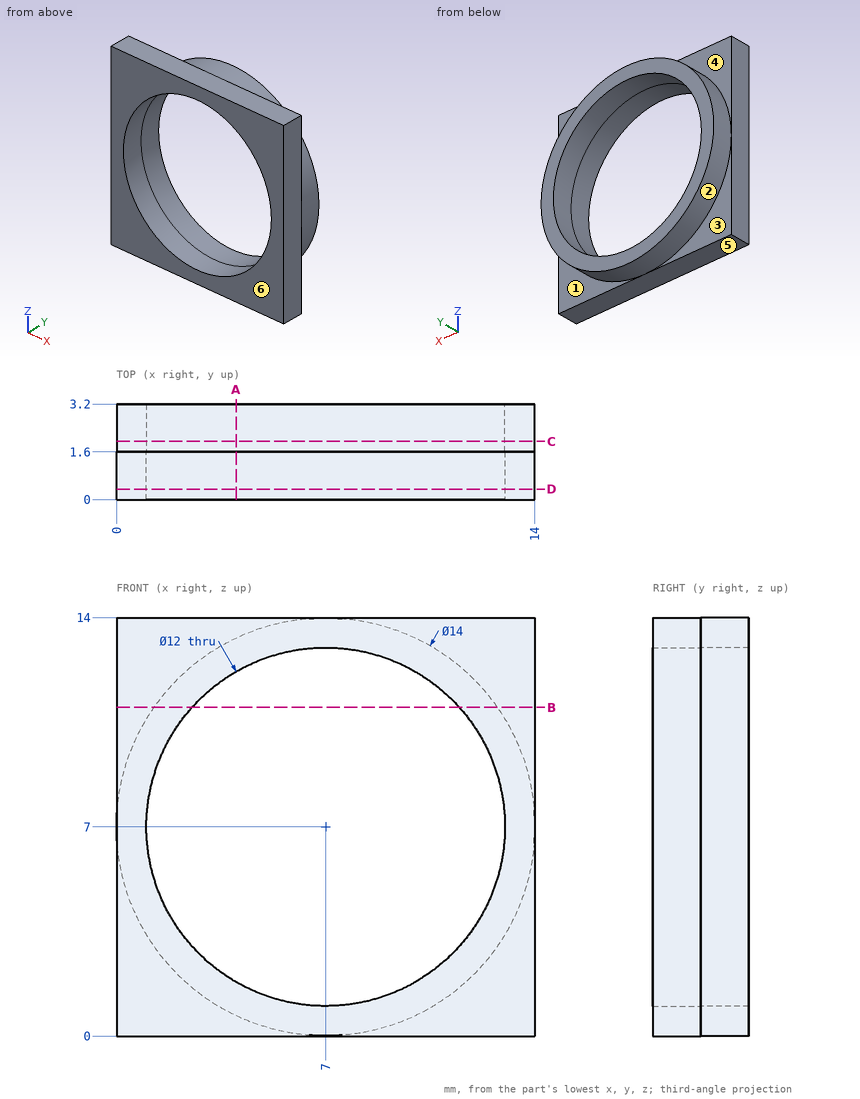
For this review, use the dimensioned drawing (mm, ordinates from the lowest corner) and the shaded views. A direction names the side the tool comes from. Coordinates: 2 decimals unless noted, no trailing zeros. Loops run counter-clockwise (first coordinate to the right, second up) from the corner with the lowest first, then second, coordinate; pieces in that order, holes last. Notation, with made-up numbers: (5, 23) - (10, 23) arc R3 ccw to (10, 28) - close; hole circle Ø3 at (53.5, -9). An arc over 180 degrees is marked (long way). Use one line per item in the form item = value. Start each with the question number.
1) Take a section at A-A (x = 4). State the section outline as (y, z) points, plus the area to 3 significant figures.
2) Take a section at D-D (y = 0.35). State the section outline as (x, z) points, plus the area to 3 significant figures.
3) Draft analysis for pull direction Y (two halves, no side actions). For the marked faces 4, 5 and 6, state which applies: released by +Y, released by -Y, zero draft, split by the parting line, or undercut.
4) For pin 1 (1 mm diameter, centred on y = 2.5, z = 8.5, fed in from -X); pin 2 (7 mm diameter, centred on x = 7, z = 7, fed in from +Y), all flat-tipped, find the tip position at first contact; note any pin that passes through.
5) Take a section at B-B (z = 11). State the section outline as (x, y) points.
6) To check wall thickness, follow probe 1 along X at (y, z) = (2.15, 7); probe 2 along Z at (x, y) = (12.25, 0.6). State the ranges of each line that lie inside material, in increasing order. Write a range as from..to.
7) Take a section at C-C (y = 1.95). State the section outline as (x, z) points.
8) For the marked faces 1, 2 and 3, list the 3-axis set-ups (+Z, -Z, +X, -X, +Y, -Y) from which the entire face can be reached by the end or side of a thin tool; tool diameter is ignored.
From the geometry:
q1.outline = (0, 0) - (1.6, 0) - (1.6, 0.68) - (3.2, 0.68) - (3.2, 1.8) - (0, 1.8) - close; (0, 12.2) - (3.2, 12.2) - (3.2, 13.32) - (1.6, 13.32) - (1.6, 14) - (0, 14) - close
q1.area = 9.38 mm2
q2.outline = (0, 0) - (14, 0) - (14, 14) - (0, 14) - close; hole circle Ø12 at (7, 7)
q2.area = 82.9 mm2
q3.face_4 = released by +Y
q3.face_5 = zero draft
q3.face_6 = released by -Y
q4.pin_1 = 0.07
q4.pin_2 = through
q5.outline = (0, 0) - (2.53, 0) - (2.53, 3.2) - (1.26, 3.2) - (1.26, 1.6) - (0, 1.6) - close; (11.47, 0) - (14, 0) - (14, 1.6) - (12.74, 1.6) - (12.74, 3.2) - (11.47, 3.2) - close
q6.probe_1 = 0..1, 13..14
q6.probe_2 = 0..4.1, 9.9..14
q7.outline = circle Ø14 at (7, 7); hole circle Ø12 at (7, 7)
q8.face_1 = -Z, +X, +Y
q8.face_2 = +Y
q8.face_3 = -Z, -X, +Y
